Check sheet for the drawn part. Datum: minimum x, y, z corner. Units: mm. A direction names the side the tool comes from. Give positions to 0.01 mm unless a question says otherwise; leave off trailing zeros. Loops run counter-clockwise (first coordinate to the right, second up) from the corner with the lowest first, then second, coordinate; pieces in that order, holes last. Notation, with made-up numbers: (57.5, 46.25) - (113.5, 46.25) arc R19 ccw to (113.5, 53.25) - close; hole circle Ø9 at (26.25, 53). An arc over 180 degrees is marked (long way). Answer in a Markdown table with one row per item.
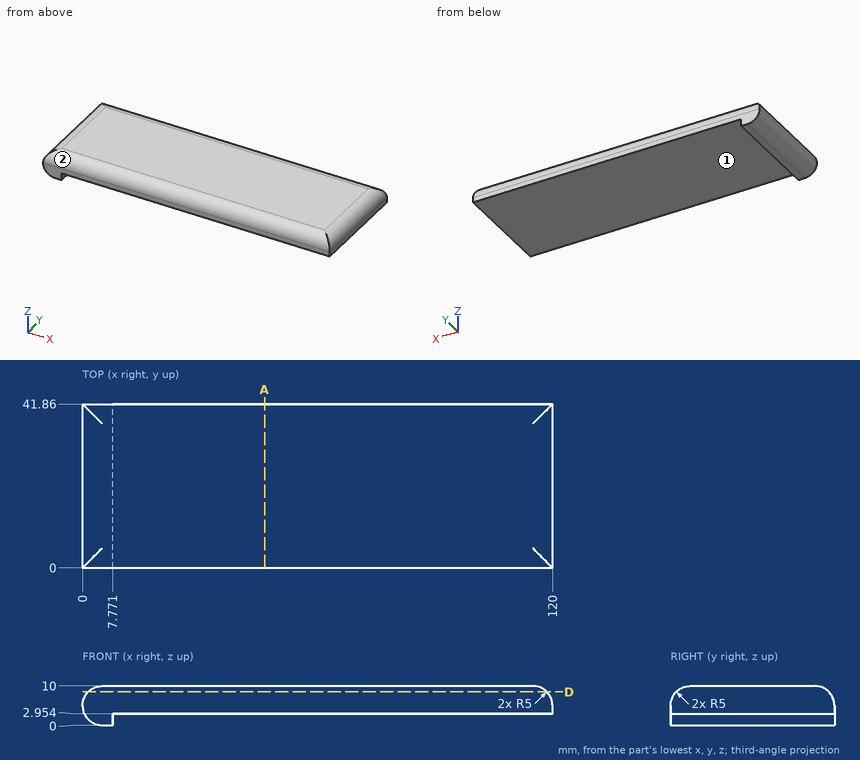
Q1. Tool access check on the marked faces 1 and 2. Record the directions out of +Z, -Z, +X, -X, +Y, -Y that give a thin tool (end or side, any length) a straight path to the whole face; none if there is none.
Completed:
| item | result |
|---|---|
| face 1 | -Z, +X, +Y, -Y |
| face 2 | +Z, +X, -X, -Y |
Q2. Sectioned sample at D-D (z = 8.5). Record the cut outline in (x, y), and give its area (3 significant figures).
Completed:
| item | result |
|---|---|
| outline | (1.43, 1.43) - (118.57, 1.43) - (118.57, 40.43) - (1.43, 40.43) - close |
| area | 4,570 mm^2 |
Q3. Sectioned sample at A-A (x = 46.5). Record the cut outline in (y, z) (1 decimal), and give its area (3 significant figures).
Completed:
| item | result |
|---|---|
| outline | (0, 3) - (41.9, 3) - (41.9, 5) arc R5 ccw to (36.9, 10) - (5, 10) arc R5 ccw to (0, 5) - close |
| area | 284 mm^2 |
Q4. Go/stop test with flat-tipped pins: P1, Ø1.5, axis at y = 21.5, z = 1.5, coming from the +X side; P2, Ø4, axis at x = 88, y = 15.5, coming from the -Z side. Record where each tip stops, or that it passes through.
Completed:
| item | result |
|---|---|
| P1 | x = 7.77 |
| P2 | z = 2.95 |
Q5. Thickness scan on line 1 (Z direction, x = 45.5, y = 24) (1 decimal); line 2 (X direction, y = 35.5, z = 5.25); line 3 (X direction, y = 14.5, z = 2.75) (1 decimal). Record the ranges inside material, lowest first.
Completed:
| item | result |
|---|---|
| line 1 | 3 to 10 |
| line 2 | 0.01 to 119.99 |
| line 3 | 0.5 to 7.8 |
